Can you work these out from the model? Positions are in its coordinate system, mm. A direction names the side the tool comes from. Coordinates: 2 decimals unless noted, no trailing zeros. Loops run counter-clockwise (first coordinate to the right, second up) from the corner with the lowest first, then second, coordinate; pieces in that order, holes last. Notation, with made-up numbers: (4.5, -36.75) -> (61.5, -36.75) arc R17 ccw to (61.5, -23.75) -> close; hole circle Ø4 at (80.5, 46). An arc over 180 degrees is marked (long way). Use one line per item in the form item = value. Start each with the question number.
(1) Thinking about a two-plate mould opening in X: for faces 1 (the flat face through (0, 0, 69)), 2 (the flat face through (15, -15, 26)), 3 (the flat face through (18.7, 18.6, 24.6)), which applies, released by +X, released by -X, zero draft, split by the parting line, or undercut?
(2) Imagine slicing it at C-C (y = 0). List the corners of the cut face in (x, z) for me.
(3) Imagine slicing it at D-D (z = 49). List the corners of the cut face in (x, y) for me.
(4) I'm going to push flat-ended pins straight in: pin 1 (1.5 mm diameter, centred on y = 18, z = 5, fed in from -X); pin 2 (2.5 mm diameter, centred on x = -15, y = 15, fed in from +Z); pin 3 (1.5 mm diameter, centred on x = 15, y = -16, fed in from +Z). Where does each tip first touch, or does it pass through?
(5) I need wall thicknesses on line 1 (Y direction, x = -15.5, z = 43.25); line 2 (Y direction, x = 15, z = 32); line 3 (Z direction, x = -7.5, y = -19). Which ranges of each line are inside material? Lowest first, please. Write a range as [from, to].
(6) On a 3-axis mill with a long thin cutter (end or side, diameter ignored), from which of +Z, -Z, +X, -X, +Y, -Y can I reach the whole of each face in a straight line? I mean faces 4 (the flat face through (21.15, 0, 25)), 5 (the cylindrical face through (-17, 15.57, 38.17)), 6 (the flat face through (7.118, 19, 5)). Say none if no direction works.
(7) Imagine slicing it at B-B (z = 9.5). List the corners of the cut face in (x, y) for me, plus the area to 3 significant figures.
(8) Imagine slicing it at A-A (x = 0). List the corners of the cut face in (y, z) for me.
```python
from build123d import *

# Parameters (mm, degrees)
BOSS_EXTRUDE1_DEPTH = 50
SKETCH2_R           = 2.5
BOSS_EXTRUDE2_DEPTH = 24
SKETCH3_R           = 1.5
CUT_EXTRUDE1_DEPTH  = 24
SKETCH4_W           = 14.23576085
SKETCH4_H           = 5.694304341
CUT_EXTRUDE2_DEPTH  = 5
SKETCH6_R           = 2.5
CUT_EXTRUDE3_DEPTH  = 5


with BuildPart() as part:
    # Sketch1 → Boss-Extrude1 (new body)
    with BuildSketch(Plane.XY):
        Polygon((-16.15, 21.15), (-21.15, 16.15), (-21.15, -16.15), (-16.15, -21.15), (16.15, -21.15), (21.15, -16.15), (21.15, 16.15), (16.15, 21.15), align=None)
    extrude(amount=BOSS_EXTRUDE1_DEPTH)

    # Sketch2 → Boss-Extrude2 (add)
    with BuildSketch(Plane.XY.offset(50)):
        Circle(SKETCH2_R)
    extrude(amount=BOSS_EXTRUDE2_DEPTH)

    # Sketch3 → Cut-Extrude1 (cut)
    with BuildSketch(Plane.XY.offset(50)):
        with Locations((-15.5, 15.5)):
            Circle(SKETCH3_R)
        with Locations((-15.5, -15.5)):
            Circle(SKETCH3_R)
        with Locations((15.5, -15.5)):
            Circle(SKETCH3_R)
        with Locations((15.5, 15.5)):
            Circle(SKETCH3_R)
    extrude(amount=-CUT_EXTRUDE1_DEPTH, mode=Mode.SUBTRACT)

    # Sketch4 → Cut-Extrude2 (cut)
    with BuildSketch(Plane(origin=(0, 21.15, 0), x_dir=(1, 0, 0), z_dir=(0, 1, 0))):
        with Locations((0, -5.299206554)):
            Rectangle(SKETCH4_W, SKETCH4_H)
    extrude(amount=-CUT_EXTRUDE2_DEPTH, mode=Mode.SUBTRACT)

    # Sketch6 → Cut-Extrude3 (cut)
    with BuildSketch(Plane.XY.offset(74)):
        Circle(SKETCH6_R)
    extrude(amount=-CUT_EXTRUDE3_DEPTH, mode=Mode.SUBTRACT)


solid = part.part
```
Worked out:
q1.face_1 = zero draft
q1.face_2 = undercut
q1.face_3 = released by +X
q2.outline = (-21.15, 0) -> (21.15, 0) -> (21.15, 50) -> (2.5, 50) -> (2.5, 69) -> (-2.5, 69) -> (-2.5, 50) -> (-21.15, 50) -> close
q3.outline = (-21.15, -16.15) -> (-16.15, -21.15) -> (16.15, -21.15) -> (21.15, -16.15) -> (21.15, 16.15) -> (16.15, 21.15) -> (-16.15, 21.15) -> (-21.15, 16.15) -> close; hole circle Ø3 at (-15.5, -15.5); hole circle Ø3 at (-15.5, 15.5); hole circle Ø3 at (15.5, -15.5); hole circle Ø3 at (15.5, 15.5)
q4.pin_1 = -20.05
q4.pin_2 = 50
q4.pin_3 = 26
q5.line_1 = [-21.15, -17], [-14, 14], [17, 21.15]
q5.line_2 = [-21.15, -16.91], [-14.09, 14.09], [16.91, 21.15]
q5.line_3 = [0, 50]
q6.face_4 = +Z, -Z, +X, +Y, -Y
q6.face_5 = +Z
q6.face_6 = +Y
q7.outline = (-21.15, -16.15) -> (-16.15, -21.15) -> (16.15, -21.15) -> (21.15, -16.15) -> (21.15, 16.15) -> (16.15, 21.15) -> (-16.15, 21.15) -> (-21.15, 16.15) -> close
q7.area = 1,740 mm2
q8.outline = (-21.15, 0) -> (21.15, 0) -> (21.15, 2.45) -> (16.15, 2.45) -> (16.15, 8.15) -> (21.15, 8.15) -> (21.15, 50) -> (2.5, 50) -> (2.5, 69) -> (-2.5, 69) -> (-2.5, 50) -> (-21.15, 50) -> close
